Verification items for the finished model (mm, model axes). Face numbers are marked on the shaded views. A direction names the side the tool comes from. Round coordinates to 2 decimals unless told otherwise and drop trailing zeros. Loops run counter-clockwise (first coordinate to the right, second up) from the corner with the lowest first, then second, coordinate; pieces in that order, holes last. Notation, with made-up numbers: (68.25, 57) -> (105.25, 57) arc R24 ccw to (105.25, 68) -> close; hole circle Ø3 at (83.25, 3). An arc over 180 degrees is marked (long way). Use CSV: the item, a comma, the result in double quotes. Start each with the question number.
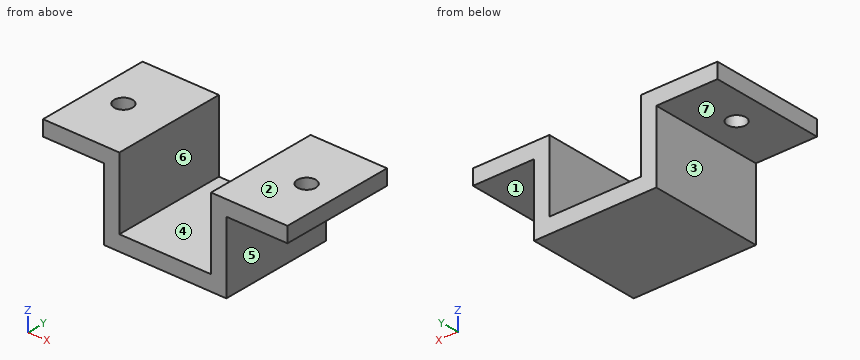
```python
from build123d import *

# Parameters (mm, degrees)
BOSS_EXTRUDE1_DEPTH = 19.05
SKETCH2_R           = 1.524
CUT_EXTRUDE1_DEPTH  = 3.54


with BuildPart() as part:
    # Sketch1 → Boss-Extrude1 (new body)
    with BuildSketch(Plane(origin=(0, 0, 0), x_dir=(1, 0, 0), z_dir=(0, 1, 0))):
        Polygon((7.62, 0), (20.32, 0), (20.32, 2.54), (10.16, 2.54), (10.16, 14.4018), (-10.16, 14.4018), (-10.16, 2.54), (-20.32, 2.54), (-20.32, 0), (-7.62, 0), (-7.62, 11.8618), (7.62, 11.8618), align=None)
    extrude(amount=BOSS_EXTRUDE1_DEPTH)

    # Sketch2 → Cut-Extrude1 (cut, through all)
    with BuildSketch(Plane(origin=(0, 0, -2.54), x_dir=(-1, 0, 0), z_dir=(0, 0, -1))):
        with Locations((15.24, 9.525)):
            Circle(SKETCH2_R)
        with Locations((-15.24, 9.525)):
            Circle(SKETCH2_R)
    extrude(amount=-CUT_EXTRUDE1_DEPTH, mode=Mode.SUBTRACT)


solid = part.part
```
Q1. Thickness scan on L1, parallel to X at y = 3.5, z = -2; L2, parallel to Y at x = 15.24, z = -1.5; L3, parallel to X at y = 11.5, z = -8.5. Record the ranges inside material, lowest first. Write a range as from..to.
Q2. Tool access check on the marked faces 1, 2, 3 and 4. Record the directions out of +Z, -Z, +X, -X, +Y, -Y that give a thin tool (end or side, any length) a straight path to the whole face; none if there is none.
Q3. Depth check by flat-ended pin: pin 1 Ø3 at (y, z) = (8.5, -10.5) entering from +X; pin 2 Ø2 at (x, y) = (-12, 5) entering from -Z; pin 3 Ø6 at (y, z) = (6.5, -3) entering from -X; pin 4 Ø1.5 at (y, z) = (13, -4.5) entering from -X. Enter the tip coordinate at first touch or a pass-through.
Q4. Cross-section at D-D (y = 16.25). Record the boundary of the cut face in (x, z), and give its area (3 significant figures).
Q5. Cross-section at B-B (z = -5.5). Record the boundary of the cut face in (x, y), and give its area (3 significant figures).
Q6. Release check for a two-part mould opening along X. For the marked faces 5, 6 and 7 record: +X half, -X half, draft (parallel to the pull), parting line (faces both ways), or undercut.
Q7. Cross-section at A-A (x = 15.24). Record the boundary of the cut face in (y, z), and give its area (3 significant figures).
Q8. Cross-section at C-C (y = 8.75). Record the boundary of the cut face in (x, z), and give its area (3 significant figures).
Answer list:
1,L1,"x = -20.32..-7.62, 7.62..20.32"
1,L2,"y = 0..8, 11.05..19.05"
1,L3,"x = -10.16..-7.62, 7.62..10.16"
2,face 1,"-Z, +X, +Y, -Y"
2,face 2,"+Z, +X, -X, +Y, -Y"
2,face 3,"-Z, -X, +Y, -Y"
2,face 4,"+Z, +Y, -Y"
3,pin 1,"stops at x = 10.16"
3,pin 2,"stops at z = -2.54"
3,pin 3,"stops at x = -20.32"
3,pin 4,"stops at x = -10.16"
4,outline,"(-20.32, -2.54) -> (-10.16, -2.54) -> (-10.16, -14.4) -> (10.16, -14.4) -> (10.16, -2.54) -> (20.32, -2.54) -> (20.32, 0) -> (7.62, 0) -> (7.62, -11.86) -> (-7.62, -11.86) -> (-7.62, 0) -> (-20.32, 0) -> close"
4,area,"163 mm2"
5,outline,"(-10.16, 0) -> (-7.62, 0) -> (-7.62, 19.05) -> (-10.16, 19.05) -> close; (7.62, 0) -> (10.16, 0) -> (10.16, 19.05) -> (7.62, 19.05) -> close"
5,area,"96.8 mm2"
6,face 5,"+X half"
6,face 6,"undercut"
6,face 7,"draft"
7,outline,"(0, -2.54) -> (8, -2.54) -> (8, 0) -> (0, 0) -> close; (11.05, -2.54) -> (19.05, -2.54) -> (19.05, 0) -> (11.05, 0) -> close"
7,area,"40.6 mm2"
8,outline,"(-20.32, -2.54) -> (-16.55, -2.54) -> (-16.55, 0) -> (-20.32, 0) -> close; (-13.93, -2.54) -> (-10.16, -2.54) -> (-10.16, -14.4) -> (10.16, -14.4) -> (10.16, -2.54) -> (13.93, -2.54) -> (13.93, 0) -> (7.62, 0) -> (7.62, -11.86) -> (-7.62, -11.86) -> (-7.62, 0) -> (-13.93, 0) -> close; (16.55, -2.54) -> (20.32, -2.54) -> (20.32, 0) -> (16.55, 0) -> close"
8,area,"150 mm2"
